Input: part model. Units: mm. Frame: model coordinates. A direction names the side the tool comes from. Coordinates: 2 decimals unless noted, no trailing zeros. Write each loop counter-clockwise with the first axis right and the second up, starting at its lowest first coordinate (ties: lowest second). Pieces come first, ordered by that corner, then holes. Notation, with made-up numbers: (32, -15) - (73, -15) arc R33 cw to (73, 24) - close; hole circle Ø8 at (-14, 68). An arc over 180 degrees is marked (long way). Use CSV: the item, a comma, the result in double quotes.
```python
from build123d import *

# Parameters (mm, degrees)
F0_W     = 118.0431097746
F0_H     = 18.2562172413
F1_DEPTH = 19.4758269936
F0_W_2   = 35.0601822138
F2_DEPTH = 101.6
F3_W     = 28.001986444
F3_H     = 42.7611395717
F4_DEPTH = 5.2572349086
F8_R     = 4.4035732841
F9_DEPTH = 109.2703565955
F10_SIZE = 2


# Not quite as in the source:
# - a feature of the source that left no trace in its solid (it failed there, or was rolled back) is left out


with BuildPart() as f1:
    # F0 (on Top) → F1 (new body)
    with BuildSketch(Plane.XY):
        with BuildLine():
            Line((76.5516459942, 9.1281086206), (76.5516459942, -9.1281086206))
            ThreePointArc((76.5516459942, -9.1281086206), (85.6797546148, 0), (76.5516459942, 9.1281086206))
        make_face()
        with Locations((17.5300911069, 0)):
            Rectangle(F0_W, F0_H)
    extrude(amount=F1_DEPTH)

    # F0 (on Top) → F2 (join)
    with BuildSketch(Plane.XY):
        with Locations((-59.0215548873, 0)):
            Rectangle(F0_W_2, F0_H)
        with BuildLine():
            ThreePointArc((-76.5516459942, 9.1281086206), (-85.6797546148, 0), (-76.5516459942, -9.1281086206))
            Line((-76.5516459942, -9.1281086206), (-76.5516459942, 9.1281086206))
        make_face()
    extrude(amount=F2_DEPTH)

    # F3 (on face) → F4 (cut)
    with BuildSketch(Plane.XZ.offset(9.1281086206)):
        with Locations((-58.9374192059, 55.1895685494)):
            Rectangle(F3_W, F3_H)
    extrude(amount=-F4_DEPTH, mode=Mode.SUBTRACT)

    # F8 (on Top) → F9 (join)
    with BuildSketch(Plane.XY):
        with Locations((76.6932368279, 0)):
            Circle(F8_R)
        with Locations((-76.5735656023, 0)):
            Circle(F8_R)
    extrude(amount=F9_DEPTH)

    # F10
    f10_edges = [f1.edges().sort_by_distance(p)[0] for p in [
        (-41.491464, -9.128109, 60.537913),
        (17.530091, -9.128109, 19.475827),
        (-41.491464, 9.128109, 60.537913),
        (85.679755, 0, 19.475827),
        (17.530091, 9.128109, 19.475827),
    ]]
    chamfer(f10_edges, length=F10_SIZE)


solid = f1.part
```
(1) Pin query (flat end, axial travel): pin 1 Ø1 at (y, z) = (5, 79.5) entering from -X; pin 2 Ø8 at (x, y) = (-32.5, 1) entering from -Z; pin 3 Ø5 at (y, z) = (6, 65) entering from +X; pin 4 Ø1.6 at (x, y) = (-64.5, -6.5) entering from +Z. Return the tip coordinate at first contact, or that it passes through.
Check values:
pin 1,"x = -84.49"
pin 2,"z = 0"
pin 3,"x = 79.37"
pin 4,"z = 101.6"
(2) Cut plane C-C on x = -56.5. Return loops of the section in (y, z), and give its area (3 significant figures).
Check values:
outline,"(-9.13, 0) - (9.13, 0) - (9.13, 101.6) - (-9.13, 101.6) - (-9.13, 76.57) - (-3.87, 76.57) - (-3.87, 33.81) - (-9.13, 33.81) - close"
area,"1,630 mm^2"
(3) Cut plane A-A on z = 48. Return loops of the section in (x, y).
Check values:
outline,"(-76.55, -9.13) - (-72.94, -9.13) - (-72.94, -3.87) - (-44.94, -3.87) - (-44.94, -9.13) - (-43.49, -9.13) - (-41.49, -7.13) - (-41.49, 7.13) - (-43.49, 9.13) - (-76.55, 9.13) arc R9.13 ccw to start; circle Ø8.81 at (76.69, 0)"
(4) Ray query, probe 1 along X at (y, z) = (0, 75.5); probe 2 along Z at (x, y) = (20, -6.5); probe 3 along X at (y, z) = (-3.75, 104). Return the intervals inside material, ascending. Write a range as from..to.
Check values:
probe 1,"-85.68..-41.49, 72.29..81.1"
probe 2,"0..19.48"
probe 3,"-78.88..-74.27, 74.38..79"
(5) Cut plane B-B on y = 0. Return loops of the section in (x, z).
Check values:
outline,"(-85.68, 0) - (85.68, 0) - (85.68, 17.48) - (83.68, 19.48) - (81.1, 19.48) - (81.1, 109.27) - (72.29, 109.27) - (72.29, 19.48) - (-41.49, 19.48) - (-41.49, 101.6) - (-72.17, 101.6) - (-72.17, 109.27) - (-80.98, 109.27) - (-80.98, 101.6) - (-85.68, 101.6) - close"
(6) Reachability of faces 5 (the flat face through (-1, 0, 0)), 6 (the flat face through (-41.491, 0, 60)), 7 (the flat face through (-72.938, -7, 55)) from +Z, -Z, +X, -X, +Y, -Y: full face, straight path, thin tool, end or side. Return the list, or none.
Check values:
face 5,"-Z, +X, -X, +Y, -Y"
face 6,"+Z, +Y, -Y"
face 7,"-Y"
(7) Draft query along X for faces 1 (the flat face through (-23, -9.128, 13)), 2 (the cylindrical face through (80.9, 1.3, 63.7)), 3 (the cylindrical face through (-72.373, 1.323, 105.381)), 4 (the conical face through (83.997, -0.164, 19.156)). Return one class per face: pulls with the +X half, pulls with the -X half, needs draft (parallel to the pull), parting line crosses it, or undercut.
Check values:
face 1,"needs draft"
face 2,"undercut"
face 3,"undercut"
face 4,"pulls with the +X half"
(8) Cut plane D-D on x = -5. Return loops of the section in (y, z), and give its area (3 significant figures).
Check values:
outline,"(-9.13, 0) - (9.13, 0) - (9.13, 17.48) - (7.13, 19.48) - (-7.13, 19.48) - (-9.13, 17.48) - close"
area,"352 mm^2"
